Could you check a few things on this model? Use its own coordinates, in mm. A direction names the side the tool comes from. Round coordinates to 2 decimals unless told otherwise and drop trailing zeros. Loops run counter-clockwise (first coordinate to the right, second up) from the corner with the lowest first, then second, coordinate; pieces in that order, holes last. Notation, with made-up numbers: (13.25, 40) -> (49.25, 40) arc R28 cw to (49.25, 69) -> close; hole circle Ø5 at (38.25, 76). An arc over 180 degrees is marked (long way). Use CSV: the item, a comma, the result in double quotes. Start each with the question number.
```python
from build123d import *

# Parameters (mm, degrees)
BOSS_EXTRUDE1_DEPTH = 6.35
SKETCH2_W           = 12.7
SKETCH2_H           = 6.35
CUT_EXTRUDE1_DEPTH  = 7.35
CUT_EXTRUDE2_DEPTH  = 7.35
CUT_EXTRUDE3_DEPTH  = 7.35


with BuildPart() as part:
    # Sketch1 → Boss-Extrude1 (new body)
    with BuildSketch(Plane.XY):
        Polygon((0, 0), (19.05, 0), (34.925, 0), (34.925, -6.35), (41.275, -6.35), (41.275, 0), (41.275, 10.795), (34.925, 10.795), (34.925, 29.845), (54.61, 29.845), (54.61, 38.735), (60.96, 38.735), (60.96, 51.435), (54.61, 51.435), (54.61, 60.325), (34.925, 60.325), (19.05, 60.325), (19.05, 66.675), (0, 66.675), (0, 60.325), (-15.875, 60.325), (-66.675, 60.325), (-66.675, 29.845), (-15.875, 29.845), (-15.875, 10.795), (-22.225, 10.795), (-22.225, 0), (-22.225, -6.35), (-15.875, -6.35), (-15.875, 0), align=None)
    extrude(amount=BOSS_EXTRUDE1_DEPTH)

    # Sketch2 → Cut-Extrude1 (cut, through all)
    with BuildSketch(Plane.XY.offset(6.35)):
        with Locations((-53.975, 33.02)):
            Rectangle(SKETCH2_W, SKETCH2_H)
    extrude(amount=-CUT_EXTRUDE1_DEPTH, mode=Mode.SUBTRACT)

    # Sketch3 → Cut-Extrude2 (cut, through all)
    with BuildSketch(Plane.XY.offset(6.35)):
        Polygon((-15.875, 21.57), (-15.875, 19.07), (-12.065, 19.07), (-12.065, 17.07), (-10.065, 17.07), (-10.065, 19.07), (-5.715, 19.07), (-5.715, 21.57), (-10.065, 21.57), (-10.065, 23.57), (-12.065, 23.57), (-12.065, 21.57), align=None)
        Polygon((34.925, 21.57), (34.925, 19.07), (31.115, 19.07), (31.115, 17.07), (29.115, 17.07), (29.115, 19.07), (24.765, 19.07), (24.765, 21.57), (29.115, 21.57), (29.115, 23.57), (31.115, 23.57), (31.115, 21.57), align=None)
    extrude(amount=-CUT_EXTRUDE2_DEPTH, mode=Mode.SUBTRACT)

    # Sketch5 → Cut-Extrude3 (cut, through all)
    with BuildSketch(Plane.XY.offset(6.35)):
        Polygon((-3.1, 56.515), (-3.1, 54.515), (-5.1, 54.515), (-5.1, 50.165), (-7.6, 50.165), (-7.6, 54.515), (-9.6, 54.515), (-9.6, 56.515), (-7.6, 56.515), (-7.6, 60.325), (-5.1, 60.325), (-5.1, 56.515), align=None)
        Polygon((-52.725, 42.005), (-50.725, 42.005), (-50.725, 40.005), (-52.725, 40.005), (-52.725, 36.195), (-55.225, 36.195), (-55.225, 40.005), (-57.225, 40.005), (-57.225, 42.005), (-55.225, 42.005), (-55.225, 46.355), (-52.725, 46.355), align=None)
        Polygon((26.65, 60.325), (26.65, 56.515), (28.65, 56.515), (28.65, 54.515), (26.65, 54.515), (26.65, 50.165), (24.15, 50.165), (24.15, 54.515), (22.15, 54.515), (22.15, 56.515), (24.15, 56.515), (24.15, 60.325), align=None)
    extrude(amount=-CUT_EXTRUDE3_DEPTH, mode=Mode.SUBTRACT)


solid = part.part
```
1. For faces 1 (the face through (22, 60.325, 3)), 2 (the face through (-22.225, 2, 3)), 3 (the face through (-5.715, 20, 3)), which set-ups out of +Z, -Z, +X, -X, +Y, -Y let a thin tool reach every point of the face, with its end or its side?
2. Suppose I cut it at A-A (y = 59). List the corners of the cut face in (x, z) for me (3 decimals), then the cut area to 3 significant figures.
3. Suppose I cut it at B-B (x = -18). List the corners of the cut face in (y, z) for me (3 decimals).
4. We'd pull the mould along X, two halves only. Please class faces 4 (the face through (58, 51.435, 3)), 5 (the face through (26.65, 58, 3)), 6 (the face through (24.765, 20, 3)): pulls with the +X half, pulls with the -X half, needs draft (parallel to the pull), parting line crosses it, or undercut.
5. Will these pins go through, and if not, where does the flat tip stop? pin 1 (0.6 mm diameter, centred on x = 30, z = 2, fed in from -Y); pin 2 (1.5 mm diameter, centred on x = 24, z = 3, fed in from +Y) (3 decimals); pin 3 (3 mm diameter, centred on y = 56.5, z = 2.5, fed in from +X).
6. Suppose I cut it at C-C (y = 32). List the corners of the cut face in (x, z) for me (3 decimals).
7. If I drill on L1, parallel to Y at x = 27, z = 2 (3 decimals); L2, parallel to Y at x = 39, z = 1.75 (3 decimals); L3, parallel to Y at x = -57, z = 3.25 (3 decimals), over which ranges is the centre line in solid material (lowest first)?
8. Suppose I cut it at D-D (x = 15). List the corners of the cut face in (y, z) for me (3 decimals).
Geometry check:
1,face 1,"+Z, -Z, +X, +Y"
1,face 2,"+Z, -Z, -X, -Y"
1,face 3,"+Z, -Z, -X"
2,outline,"(-66.675, 0) -> (-7.6, 0) -> (-7.6, 6.35) -> (-66.675, 6.35) -> close; (-5.1, 0) -> (24.15, 0) -> (24.15, 6.35) -> (-5.1, 6.35) -> close; (26.65, 0) -> (54.61, 0) -> (54.61, 6.35) -> (26.65, 6.35) -> close"
2,area,"738 mm²"
3,outline,"(-6.35, 0) -> (10.795, 0) -> (10.795, 6.35) -> (-6.35, 6.35) -> close; (29.845, 0) -> (60.325, 0) -> (60.325, 6.35) -> (29.845, 6.35) -> close"
4,face 4,"needs draft"
4,face 5,"undercut"
4,face 6,"pulls with the +X half"
5,pin 1,"stops at y = 0"
5,pin 2,"stops at y = 60.325"
5,pin 3,"stops at x = 54.61"
6,outline,"(-66.675, 0) -> (-60.325, 0) -> (-60.325, 6.35) -> (-66.675, 6.35) -> close; (-47.625, 0) -> (54.61, 0) -> (54.61, 6.35) -> (-47.625, 6.35) -> close"
7,L1,"y = 0 to 19.07, 21.57 to 54.515, 56.515 to 60.325"
7,L2,"y = -6.35 to 10.795, 29.845 to 60.325"
7,L3,"y = 36.195 to 40.005, 42.005 to 60.325"
8,outline,"(0, 0) -> (66.675, 0) -> (66.675, 6.35) -> (0, 6.35) -> close"
